The model under review builds one solid part; all positions refer to its coordinate system, in mm. A direction names the side the tool comes from. Round coordinates to 2 decimals unless told otherwise and drop trailing zeros. Write each loop counter-clockwise with the first axis right and the second up, starting at its lowest first coordinate (ties: lowest second). Pieces come first, ordered by that corner, then holes. Notation, with made-up numbers: (-33.5, -33.75) -> (-8.5, -33.75) arc R18 cw to (-8.5, -15.75) -> close; hole circle Ø10 at (-3, -24.75). An arc over 180 degrees is marked (long way). Answer as a JSON object with one key per item and string values. Group by question number.
1) We need section A-A, the plane x = -21.25. Write out the cut boundary in (y, z).
2) Mouldability with a two-part tool opening along Z and no side actions: class faces 1 (the flat face through (-18, -29, -2)), 2 (the conical face through (-17.702, -29.863, 0.36)), 3 (the flat face through (-18, -29, 3)), 4 (the cylindrical face through (-13.51, -29.41, 0.54)) as pulls with the +Z half, pulls with the -Z half, needs draft (parallel to the pull), parting line crosses it, or undercut.
3) We need section D-D, the plane z = 0.85. Count the separate pieces of the cut face and the enclosed holes in it, then the cut area to 3 significant figures.
4) We need section B-B, the plane z = -1.45. Write out the cut boundary in (x, y).
5) Machinability: for faces 5 (the flat face through (-16, -33.608, 0)), 6 (the cylindrical face through (-16.435, -32.087, 0.305)), which of the approach directions +Z, -Z, +X, -X, +Y, -Y give a long, thin tool a straight path to every point of the face, cutting with its end or side? Answer none if there is none.
6) Insertion check: pin 1 Ø2.5 at (x, z) = (-17.92, 0.5) entering from -Y. The pin has a flat end and moves straight along its axis. Give the tip position at first contact, or say it passes through.
7) We need section C-C, the plane y = -32. Write out the cut boundary in (x, z), then the cut area to 3 significant figures.
8) To check wall thickness, follow probe 1 along X at (y, z) = (-33, 0.5); probe 2 along X at (y, z) = (-28.75, 2.5); probe 3 along Z at (x, y) = (-19.25, -31.25). State the ranges of each line that lie inside material, in increasing order. Write a range as [from, to].
from build123d import *

# Parameters (mm, degrees)
BOSS_EXTRU_1_DEPTH      = 3
BOSS_EXTRU_1_DEPTH_BACK = 2
ESQUISSE1_W             = 15
ESQUISSE1_H             = 10
D_GAGEMENT_M1_61_D      = 1.8
D_GAGEMENT_M1_61_DEPTH  = 28.17
D_GAGEMENT_M1_61_TIP    = 0.540774557
D_GAGEMENT_M1_62_D      = 3
D_GAGEMENT_M1_62_DEPTH  = 3
D_GAGEMENT_M1_62_TIP    = 0.901290929


with BuildPart() as part:
    # Esquisse1 → Boss.-Extru.1 (new, two sides: drawn at the far end of the back side and taken through both)
    with BuildSketch(Plane.XY.offset(-BOSS_EXTRU_1_DEPTH_BACK)):
        with Locations((-17.922006263, -28.608262445)):
            Rectangle(ESQUISSE1_W, ESQUISSE1_H)
    extrude(amount=BOSS_EXTRU_1_DEPTH + BOSS_EXTRU_1_DEPTH_BACK)

    # Dégagement M1.61
    with Locations(Plane(origin=(-21.922006263, -28.608262445, -2), x_dir=(-1, 0, 0), z_dir=(0, 0, -1))):
        with Locations((0, 0), (-8, 0)):
            Hole(D_GAGEMENT_M1_61_D / 2, depth=D_GAGEMENT_M1_61_DEPTH)
            with Locations((0, 0, -(D_GAGEMENT_M1_61_DEPTH + D_GAGEMENT_M1_61_TIP / 2))):  # 118° drill point
                Cone(0, D_GAGEMENT_M1_61_D / 2, D_GAGEMENT_M1_61_TIP, mode=Mode.SUBTRACT)

    # Dégagement M1.62
    with Locations(Plane(origin=(-17.922006263, -33.608262445, 0.5), x_dir=(0, 0, -1), z_dir=(0, -1, 0))):
        with Locations((0, 0)):
            Hole(D_GAGEMENT_M1_62_D / 2, depth=D_GAGEMENT_M1_62_DEPTH)
            with Locations((0, 0, -(D_GAGEMENT_M1_62_DEPTH + D_GAGEMENT_M1_62_TIP / 2))):  # 118° drill point
                Cone(0, D_GAGEMENT_M1_62_D / 2, D_GAGEMENT_M1_62_TIP, mode=Mode.SUBTRACT)


solid = part.part
Here are the results:
{
 "1": {"outline": "(-33.61, -2) -> (-29.21, -2) -> (-29.21, 3) -> (-33.61, 3) -> close; (-28.01, -2) -> (-23.61, -2) -> (-23.61, 3) -> (-28.01, 3) -> close"},
 "2": {"face 1": "pulls with the -Z half", "face 2": "undercut", "face 3": "pulls with the +Z half", "face 4": "needs draft"},
 "3": {"separate pieces": "1", "enclosed holes": "2", "area": "135 mm^2"},
 "4": {"outline": "(-25.42, -33.61) -> (-10.42, -33.61) -> (-10.42, -23.61) -> (-25.42, -23.61) -> close; hole circle Ø1.8 at (-21.92, -28.61); hole circle Ø1.8 at (-13.92, -28.61)"},
 "5": {"face 5": "+Z, -Z, +X, -X, -Y", "face 6": "-Y"},
 "6": {"pin 1": "stops at y = -30.46"},
 "7": {"outline": "(-25.42, -2) -> (-10.42, -2) -> (-10.42, 3) -> (-25.42, 3) -> close; hole circle Ø3 at (-17.92, 0.5)", "area": "67.9 mm^2"},
 "8": {"probe 1": "x = [-25.42, -19.42], [-16.42, -10.42]", "probe 2": "x = [-25.42, -22.81], [-21.03, -14.81], [-13.03, -10.42]", "probe 3": "z = [-2, -0.2], [1.2, 3]"}
}
